Input: part model. Units: mm. Frame: model coordinates. A direction names the side the tool comes from. Give positions to 0.01 mm unless a question says otherwise; leave off trailing zeros. Loops run counter-clockwise (first coordinate to the right, second up) from the corner with the lowest first, then second, coordinate; pieces in that order, holes last.
from build123d import *

# Parameters (mm, degrees)
F1_DEPTH = 80
F3_DEPTH = 27.9
F4_R     = 20
F6_R     = 39.99999
F7_R     = 5
F8_DEPTH = 148.2


# Not quite as in the source:
# - a fillet or chamfer is up to 0.001 mm smaller than in the source, because OpenCascade refuses the exact size


with BuildPart() as f1:
    # F0 (on Front) → F1 (new body)
    with BuildSketch(Plane.XZ):
        Polygon((-150, 0), (0, 0), (0, 10), (-109.5854811567, 10), (-155.3589838486, 89.2820323028), (-164.0192378865, 84.2820323028), (-134.0192378865, 32.3205080757), (-151.3397459622, 22.3205080757), (-181.3397459622, 74.2820323028), (-190, 69.2820323028), align=None)
    extrude(amount=F1_DEPTH)

    # F2 (on Top) → F3 (cut)
    with BuildSketch(Plane.XY):
        with BuildLine():
            Line((-60, -40), (-60, -30))
            ThreePointArc((-60, -30), (-70, -40), (-60, -50))
            Line((-60, -50), (-60, -40))
        make_face()
        with BuildLine():
            ThreePointArc((-50, -40), (-52.9289321881, -32.9289321881), (-60, -30))
            Line((-60, -30), (-60, -40))
            Line((-60, -40), (-50, -40))
        make_face()
        with BuildLine():
            ThreePointArc((-60, -50), (-52.9289321881, -47.0710678119), (-50, -40))
            Line((-50, -40), (-60, -40))
            Line((-60, -40), (-60, -50))
        make_face()
        with BuildLine():
            Line((0, -50), (0, -40))
            Line((0, -40), (-50, -40))
            ThreePointArc((-50, -40), (-52.9289321881, -47.0710678119), (-60, -50))
            Line((-60, -50), (0, -50))
        make_face()
        with BuildLine():
            Line((0, -40), (0, -30))
            Line((0, -30), (-60, -30))
            ThreePointArc((-60, -30), (-52.9289321881, -32.9289321881), (-50, -40))
            Line((-50, -40), (0, -40))
        make_face()
    extrude(amount=F3_DEPTH, mode=Mode.SUBTRACT)

    # F4
    f4_edges = [f1.edges().sort_by_distance(p)[0] for p in [
        (0, 0, 5),
        (0, -80, 5),
    ]]
    fillet(f4_edges, radius=F4_R)

    # F6 (radius 40 in the source; OpenCascade refuses exactly that, so slightly less here)
    f6_edges = [f1.edges().sort_by_distance(p)[0] for p in [
        (-159.689111, 0, 86.782032),
        (-185.669873, 0, 71.782032),
        (-185.669873, -80, 71.782032),
        (-159.689111, -80, 86.782032),
    ]]
    fillet(f6_edges, radius=F6_R)

    # F7
    f7_edges = [f1.edges().sort_by_distance(p)[0] for p in [
        (-109.585481, -40, 10),
    ]]
    fillet(f7_edges, radius=F7_R)

    # F5 (on face) → F8 (cut)
    with BuildSketch(Plane(origin=(-77.8589838486, 0, -44.9519052838), x_dir=(0, 1, 0), z_dir=(0.8660254038, 0, 0.5))):
        with BuildLine():
            Line((-40, 112.1529946162), (-40, 102.1529946162))
            ThreePointArc((-40, 102.1529946162), (-32.9289321881, 105.0819268043), (-30, 112.1529946162))
            ThreePointArc((-30, 112.1529946162), (-40, 122.1529946162), (-50, 112.1529946162))
            Line((-50, 112.1529946162), (-40, 112.1529946162))
        make_face()
        with BuildLine():
            ThreePointArc((-50, 112.1529946162), (-47.0710678119, 105.0819268043), (-40, 102.1529946162))
            Line((-40, 102.1529946162), (-40, 112.1529946162))
            Line((-40, 112.1529946162), (-50, 112.1529946162))
        make_face()
    extrude(amount=-F8_DEPTH, mode=Mode.SUBTRACT)


solid = f1.part
(1) Cut plane B-B (y = -33). Return the cut outline in (x, z).
Values follow:
outline: (-189.69, 68.75) - (-172.15, 38.36) - (-163.49, 43.36) - (-181.03, 73.75) - close; (-165.01, 25.99) - (-150, 0) - (-67.14, 0) - (-67.14, 10) - (-106.7, 10) arc R5 cw to (-111.03, 12.5) - (-130.36, 45.99) - (-139.03, 40.99) - (-134.02, 32.32) - (-151.34, 22.32) - (-156.35, 30.99) - close; (-163.71, 83.75) - (-146.17, 53.36) - (-137.51, 58.36) - (-155.05, 88.75) - close
(2) Cut plane D-D (y = -5.5). Return the cut outline in (x, z).
Values follow:
outline: (-180.12, 52.17) - (-150, 0) - (-6.23, 0) - (-6.23, 10) - (-106.7, 10) arc R5 cw to (-111.03, 12.5) - (-145.48, 72.17) - (-154.14, 67.17) - (-134.02, 32.32) - (-151.34, 22.32) - (-171.46, 57.17) - close
(3) Reachability of faces 1 (the flat face through (-142.56, -39.44, 27.39)), 2 (the flat face through (-64.5, -30.6, 10)), 3 (the flat face through (-30, -30, 5)), 4 (the flat face through (0, -25, 5)) from +Z, -Z, +X, -X, +Y, -Y: full face, straight path, thin tool, end or side. Return the list, or none.
Values follow:
face 1: +Y, -Y
face 2: +Z, +X, +Y, -Y
face 3: +Z, -Z, +X
face 4: +Z, -Z, +X, +Y, -Y
(4) Cut plane A-A (x = -36). Return the cut outline in (y, z), and give its area (3 significant figures).
Values follow:
outline: (-80, 0) - (-50, 0) - (-50, 10) - (-80, 10) - close; (-30, 0) - (0, 0) - (0, 10) - (-30, 10) - close
area: 600 mm2
(5) Cut plane C-C (y = -44). Return the cut outline in (x, z).
Values follow:
outline: (-189.9, 69.11) - (-173.16, 40.11) - (-164.5, 45.11) - (-181.24, 74.11) - close; (-163.99, 24.24) - (-150, 0) - (-69.17, 0) - (-69.17, 10) - (-106.7, 10) arc R5 cw to (-111.03, 12.5) - (-129.35, 44.24) - (-138.01, 39.24) - (-134.02, 32.32) - (-151.34, 22.32) - (-155.33, 29.24) - close; (-163.92, 84.11) - (-147.18, 55.11) - (-138.52, 60.11) - (-155.26, 89.11) - close
(6) Pin query (flat end, axial travel): pin 1 Ø11 at (x, z) = (-17, 7) entering from -Y; pin 2 Ø2 at (x, y) = (-96, -40) entering from +Z; pin 3 Ø1.5 at (y, z) = (-32, 28) entering from -X; pin 4 Ø4 at (y, z) = (-63.5, 35) entering from -X. Return the tip coordinate at first contact, or that it passes through.
Values follow:
pin 1: stops at y = -80
pin 2: stops at z = 10
pin 3: stops at x = -166.16
pin 4: stops at x = -171.36
(7) Mould query, pull axis X, two halves, no side actions, for faces 5 (the flat face through (-112, 0, 11)), 6 (the flat face through (-149.23, -39.44, 58.67)), 7 (the flat face through (0, -55, 5)). Classes: +X half, -X half, draft (parallel to the pull), parting line (faces both ways), or undercut.
Values follow:
face 5: draft
face 6: undercut
face 7: +X half
(8) Ray query, probe 1 along Z at (x, y) = (-106, -24.5); probe 2 along X at (y, z) = (-13.5, 27.5); probe 3 along Z at (x, y) = (-137, -13). Return the intervals inside material, ascending.
Values follow:
probe 1: z = 0 to 10
probe 2: x = -165.88 to -154.33, -142.37 to -119.69
probe 3: z = 0 to 30.6, 37.48 to 57.48
